Verification items for the finished model (mm, model axes). Face numbers are marked on the shaded views. A direction names the side the tool comes from. Coordinates: 2 decimals unless noted, no trailing zeros. Write each loop counter-clockwise with the first axis right and the second up, starting at its lowest first coordinate (ties: lowest second). Pieces come first, ordered by that corner, then holes. Notation, with made-up numbers: M 78,49.25 L 83,49.25 A28 cw 83,83.25 Z; hole C -5,74.25 d11. An arc over 180 degrees is marked long. Answer in a Markdown table with one row per item.
from build123d import *

# Parameters (mm, degrees)
BOSS_EXTRUDE1_DEPTH = 60
SKETCH2_R           = 2.75
CUT_EXTRUDE1_DEPTH  = 107.963778916


with BuildPart() as part:
    # Sketch1 → Boss-Extrude1 (new, symmetric)
    with BuildSketch(Plane.YZ):
        Polygon((39, 0), (39, 54.5), (0, 54.5), (0, 79.5), (5, 79.5), (5, 59.5), (44, 59.5), (44, 0), (44, -59.5), (5, -59.5), (5, -79.5), (0, -79.5), (0, -54.5), (39, -54.5), align=None)
    extrude(amount=BOSS_EXTRUDE1_DEPTH, both=True)

    # Sketch2 → Cut-Extrude1 (cut, through all)
    with BuildSketch(Plane(origin=(0, 5, 0), x_dir=(-1, 0, 0), z_dir=(0, 1, 0))):
        with Locations(Location((-45.72, 68.58, 0), (0, 0, 90))):
            Circle(SKETCH2_R)
        with Locations(Location((45.72, 68.58, 0), (0, 0, 90))):
            Circle(SKETCH2_R)
        with Locations(Location((45.72, -68.58, 0), (0, 0, 90))):
            Circle(SKETCH2_R)
        with Locations(Location((-45.72, -68.58, 0), (0, 0, 90))):
            Circle(SKETCH2_R)
    extrude(amount=-CUT_EXTRUDE1_DEPTH, mode=Mode.SUBTRACT)


solid = part.part
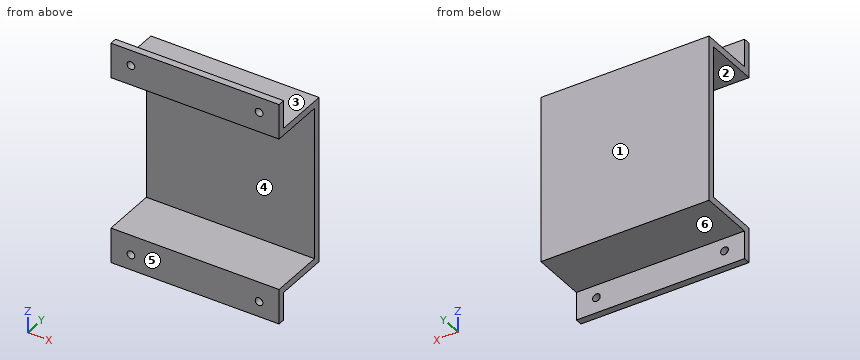
1) Depth check by flat-ended pin: pin 1 (6 mm diameter, centred on x = -24, z = -73.5, fed in from +Y); pin 2 (11.5 mm diameter, centred on x = -26, y = 21, fed in from +Z); pin 3 (4 mm diameter, centred on x = -35.5, y = 22, fed in from -Z). Enter the tip coordinate at first touch or a pass-through.
Response values:
| item | result |
|---|---|
| pin 1 | stops at y = 5 |
| pin 2 | stops at z = 59.5 |
| pin 3 | stops at z = -59.5 |
2) Sectioned sample at B-B (y = 19). Record the cut outline in (x, z).
Response values:
| item | result |
|---|---|
| outline | M -60,-59.5 L 60,-59.5 L 60,-54.5 L -60,-54.5 Z; M -60,54.5 L 60,54.5 L 60,59.5 L -60,59.5 Z |
3) Thickness scan on L1, parallel to X at y = 2.35, z = -68.58; L2, parallel to Z at x = -2, y = 12.5; L3, parallel to X at y = 1, z = 68. Record the ranges inside material, lowest first. Write a range as [from, to].
Response values:
| item | result |
|---|---|
| L1 | x = [-60, -48.47], [-42.97, 42.97], [48.47, 60] |
| L2 | z = [-59.5, -54.5], [54.5, 59.5] |
| L3 | x = [-60, -48.41], [-43.03, 43.03], [48.41, 60] |
4) Sectioned sample at C-C (z = 68.58). Record the cut outline in (x, y), then the cut area to 3 significant figures.
Response values:
| item | result |
|---|---|
| outline | M -60,0 L -48.47,0 L -48.47,5 L -60,5 Z; M -42.97,0 L 42.97,0 L 42.97,5 L -42.97,5 Z; M 48.47,0 L 60,0 L 60,5 L 48.47,5 Z |
| area | 545 mm² |
5) Sectioned sample at D-D (x = -10.5). Record the cut outline in (y, z), then the cut area to 4 significant figures.
Response values:
| item | result |
|---|---|
| outline | M 0,-79.5 L 5,-79.5 L 5,-59.5 L 44,-59.5 L 44,59.5 L 5,59.5 L 5,79.5 L 0,79.5 L 0,54.5 L 39,54.5 L 39,-54.5 L 0,-54.5 Z |
| area | 1,185 mm² |
6) Tool access check on the marked faces 4, 5 and 6. Record the directions out of +Z, -Z, +X, -X, +Y, -Y that give a thin tool (end or side, any length) a straight path to the whole face; none if there is none.
Response values:
| item | result |
|---|---|
| face 4 | +X, -X, -Y |
| face 5 | +Z, -Z, +X, -X, -Y |
| face 6 | -Z, +X, -X, +Y |
7) Release check for a two-part mould opening along Z. For the marked faces 1, 2 and 3 record: +Z half, -Z half, draft (parallel to the pull), parting line (faces both ways), or undercut.
Response values:
| item | result |
|---|---|
| face 1 | draft |
| face 2 | undercut |
| face 3 | +Z half |
8) Sectioned sample at A-A (x = -45.72). Record the cut outline in (y, z), then the cut area to 3 significant figures.
Response values:
| item | result |
|---|---|
| outline | M 0,-79.5 L 5,-79.5 L 5,-71.33 L 0,-71.33 Z; M 0,-65.83 L 5,-65.83 L 5,-59.5 L 44,-59.5 L 44,59.5 L 5,59.5 L 5,65.83 L 0,65.83 L 0,54.5 L 39,54.5 L 39,-54.5 L 0,-54.5 Z; M 0,71.33 L 5,71.33 L 5,79.5 L 0,79.5 Z |
| area | 1,130 mm² |
